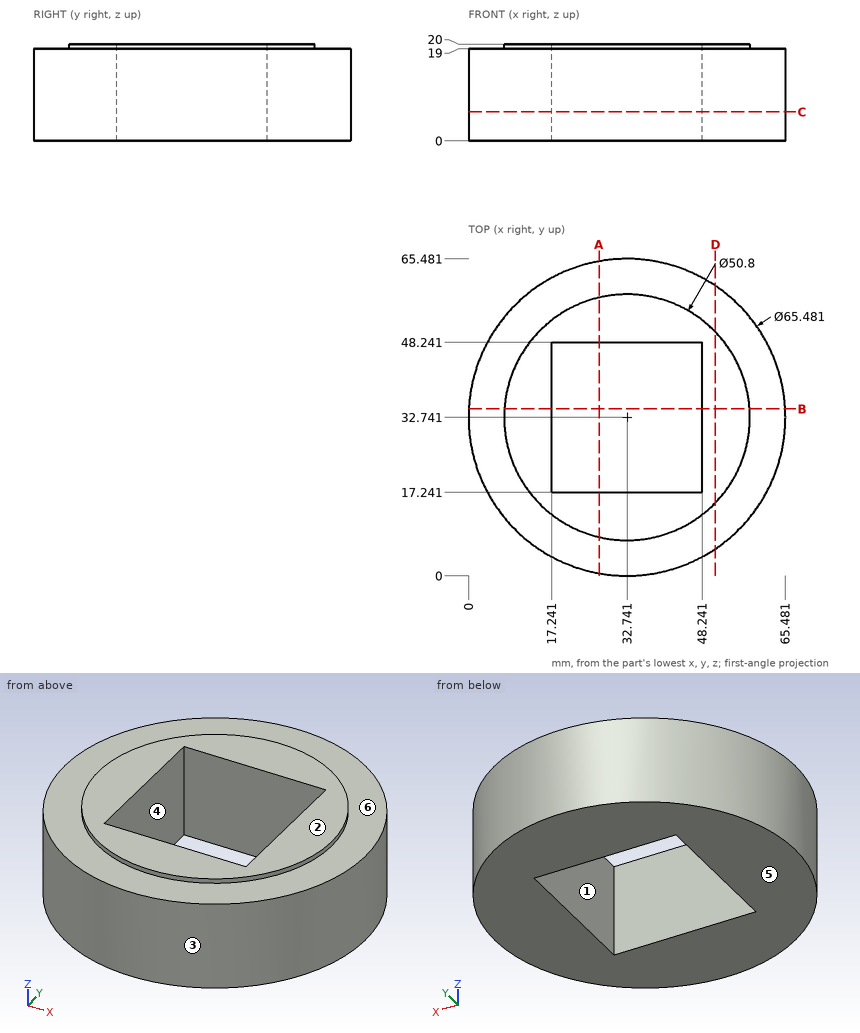
For this review, use the dimensioned drawing (mm, ordinates from the lowest corner) and the shaded views. A direction names the side the tool comes from. Round coordinates to 2 decimals unless told otherwise and drop trailing zeros. Write each loop counter-clockwise with the first axis right and the second up, starting at its lowest first coordinate (ties: lowest second). Pieces come first, ordered by that corner, then holes. Notation, with made-up numbers: (64.5, -38) -> (120.5, -38) arc R19 ccw to (120.5, -5) -> close; hole circle Ø8 at (30, -28.5). An arc over 180 degrees is marked (long way). Answer in a Markdown table with one row per item.
Q1. Take a section at A-A, the plane x = 27. State the section outline as (y, z) points.
The answers:
| item | result |
|---|---|
| outline | (0.51, 0) -> (17.24, 0) -> (17.24, 20) -> (8, 20) -> (8, 19) -> (0.51, 19) -> close; (48.24, 0) -> (64.97, 0) -> (64.97, 19) -> (57.48, 19) -> (57.48, 20) -> (48.24, 20) -> close |
Q2. Clearance check with flat-ended pins moving along their axes: pin 1 Ø12 at (y, z) = (22.5, 15.5) entering from -X; pin 2 Ø6 at (x, z) = (28.5, 18) entering from -Y; pin 3 Ø3 at (y, z) = (8.5, 10) entering from +X (1 decimal). State where each tip first meets the part, or that it passes through.
The answers:
| item | result |
|---|---|
| pin 1 | x = 0.28 |
| pin 2 | y = 0.02 |
| pin 3 | x = 56.3 |
Q3. Take a section at C-C, the plane z = 6. State the section outline as (x, y) points, then the cut area to 3 significant figures.
The answers:
| item | result |
|---|---|
| outline | circle Ø65.48 at (32.74, 32.74); hole (17.24, 17.24) -> (48.24, 17.24) -> (48.24, 48.24) -> (17.24, 48.24) -> close |
| area | 2,410 mm² |
Q4. For the marked faces 4, 5 and 6, list the 3-axis set-ups (+Z, -Z, +X, -X, +Y, -Y) from which the entire face can be reached by the end or side of a thin tool; tool diameter is ignored.
The answers:
| item | result |
|---|---|
| face 4 | +Z, -Z |
| face 5 | -Z, +X, -X, +Y, -Y |
| face 6 | +Z |
Q5. Draft analysis for pull direction Y (two halves, no side actions). For the marked faces 1, 2 and 3, state which applies: +Y half, -Y half, draft (parallel to the pull), parting line (faces both ways), or undercut.
The answers:
| item | result |
|---|---|
| face 1 | undercut |
| face 2 | draft |
| face 3 | parting line |
Q6. Take a section at D-D, the plane x = 51. State the section outline as (y, z) points (1 decimal), then the cut area to 3 significant figures.
The answers:
| item | result |
|---|---|
| outline | (5.6, 0) -> (59.9, 0) -> (59.9, 19) -> (50.4, 19) -> (50.4, 20) -> (15.1, 20) -> (15.1, 19) -> (5.6, 19) -> close |
| area | 1,070 mm² |
Q7. To check wall thickness, follow L1, parallel to Y at x = 33.5, z = 15.75; L2, parallel to X at y = 17.5, z = 2.5 (1 decimal). State the ranges of each line that lie inside material, in increasing order. Write a range as [from, to].
The answers:
| item | result |
|---|---|
| L1 | [0.01, 17.24], [48.24, 65.47] |
| L2 | [3.8, 17.2], [48.2, 61.7] |
Q8. Take a section at B-B, the plane y = 34.5. State the section outline as (x, z) points.
The answers:
| item | result |
|---|---|
| outline | (0.05, 0) -> (17.24, 0) -> (17.24, 20) -> (7.4, 20) -> (7.4, 19) -> (0.05, 19) -> close; (48.24, 0) -> (65.43, 0) -> (65.43, 19) -> (58.08, 19) -> (58.08, 20) -> (48.24, 20) -> close |
